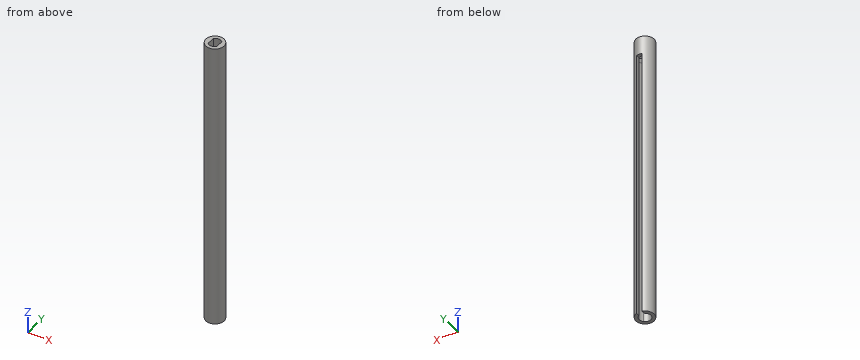
from build123d import *

# Parameters (mm, degrees)
SKETCH1_R           = 5
SKETCH1_R_2         = 3.2
BOSS_EXTRUDE1_DEPTH = 160
CUT_EXTRUDE1_DEPTH  = 150
FILLET1_R           = 5


with BuildPart() as part:
    # Sketch1 → Boss-Extrude1 (new body)
    # profile 1 of 3: a face of its own
    with BuildSketch(Plane.XY):
        Circle(SKETCH1_R)
        Circle(SKETCH1_R_2, mode=Mode.SUBTRACT)
    # profile 2 of 3: a face of its own
    with BuildSketch(Plane.XY):
        with BuildLine():
            ThreePointArc((3.2, 0), (2.979932885, 1.166190379), (2.35, 2.171980663))
            Line((2.35, 2.171980663), (2.35, -2.171980663))
            ThreePointArc((2.35, -2.171980663), (2.979932885, -1.166190379), (3.2, 0))
        make_face()
    # profile 3 of 3: a face of its own
    with BuildSketch(Plane.XY):
        with BuildLine():
            Line((-2.35, -2.171980663), (-2.35, 2.171980663))
            ThreePointArc((-2.35, 2.171980663), (-3.2, 0), (-2.35, -2.171980663))
        make_face()
    extrude(amount=BOSS_EXTRUDE1_DEPTH)

    # Sketch2 → Cut-Extrude1 (cut)
    with BuildSketch(Plane.XY):
        with BuildLine():
            Line((1.5, 0), (1.5, -2.826658805))
            ThreePointArc((1.5, -2.826658805), (2.74226184, -1.64924225), (3.2, 0))
            ThreePointArc((3.2, 0), (2.74226184, 1.64924225), (1.5, 2.826658805))
            Line((1.5, 2.826658805), (1.5, 0))
        make_face()
        with BuildLine():
            ThreePointArc((-1.5, 2.826658805), (0, 3.2), (1.5, 2.826658805))
            Line((1.5, 2.826658805), (1.5, 5))
            Line((1.5, 5), (-1.5, 5))
            Line((-1.5, 5), (-1.5, 2.826658805))
        make_face()
        with BuildLine():
            ThreePointArc((-1.5, 2.826658805), (-3.2, 0), (-1.5, -2.826658805))
            Line((-1.5, -2.826658805), (-1.5, 0))
            Line((-1.5, 0), (-1.5, 2.826658805))
        make_face()
    extrude(amount=CUT_EXTRUDE1_DEPTH, mode=Mode.SUBTRACT)

    # Fillet1
    # the kernel refuses this fillet: 5 mm, written as the material it takes off along each edge
    with BuildSketch(Plane(origin=(2.35, 14.671980663, 150), x_dir=(0, 0, 1), z_dir=(0, -1, 0))) as fillet1_piece_1_section:
        with BuildLine():
            CenterArc((FILLET1_R, -FILLET1_R), FILLET1_R, 90, 90)
            Line((0, -FILLET1_R), (0, 0))
            Line((0, 0), (FILLET1_R, 0))
        make_face()
    fillet1_piece_1 = extrude(amount=29.343961326, mode=Mode.PRIVATE)
    fillet1_piece_1 = fillet1_piece_1 & Plane(origin=(0, 0, 151.715946683), x_dir=(1, 0, 0), z_dir=(0, 0, -1)) * Cylinder(3.2, 79, mode=Mode.PRIVATE)
    add(fillet1_piece_1, mode=Mode.SUBTRACT)
    with BuildSketch(Plane(origin=(-2.35, -14.671980663, 150), x_dir=(-1, 0, 0), z_dir=(0, 1, 0))) as fillet1_piece_2_section:
        with BuildLine():
            CenterArc((FILLET1_R, FILLET1_R), FILLET1_R, 180, 90)
            Line((0, FILLET1_R), (0, 0))
            Line((0, 0), (FILLET1_R, 0))
        make_face()
    fillet1_piece_2 = extrude(amount=29.343961326, mode=Mode.PRIVATE)
    fillet1_piece_2 = fillet1_piece_2 & Plane(origin=(0, 0, 151.715946769), x_dir=(1, 0, 0), z_dir=(0, 0, -1)) * Cylinder(3.2, 79, mode=Mode.PRIVATE)
    add(fillet1_piece_2, mode=Mode.SUBTRACT)


solid = part.part
Verification items for the finished model (mm, model axes). Round coordinates to 2 decimals unless told otherwise and drop trailing zeros. Order: outer loops, then holes, each group sorted by start corner. A loop starts at its lowest first (then second) coordinate and runs counter-clockwise, first axis right, second up.
1. Section check A-A on x = 0. Record the cut outline in (y, z), then the cut area to 3 significant figures.
Final values:
outline: (-5, 0) - (-3.2, 0) - (-3.2, 160) - (-5, 160) - close; (3.2, 150) - (5, 150) - (5, 160) - (3.2, 160) - close
area: 306 mm2
2. Thickness scan on L1, parallel to X at y = -4.5, z = 55; L2, parallel to X at y = 0.5, z = 137; L3, parallel to X at y = 1.25, z = 97.5. Record the ranges inside material, lowest first.
Final values:
L1: x = -2.18 to 2.18
L2: x = -4.97 to -3.16, 3.16 to 4.97
L3: x = -4.84 to -2.95, 2.95 to 4.84
3. Go/stop test with flat-tipped pins: P1, Ø0.7, axis at x = 0.5, y = 3.5, coming from the -Z side; P2, Ø1.5, axis at x = 1.5, z = 143.5, coming from the -Y side; P3, Ø1, axis at y = 4, z = 123.5, coming from the +X side. Record where each tip stops, or that it passes through.
Final values:
P1: stops at z = 150
P2: stops at y = -4.94
P3: stops at x = 3.57
4. Section check B-B on z = 38.5. Record the cut outline in (x, y), then the cut area to 3 significant figures.
Final values:
outline: (-1.5, 2.83) - (-1.5, 4.77) arc R5 ccw (long way) to (1.5, 4.77) - (1.5, 2.83) arc R3.2 cw (long way) to start
area: 40.8 mm2
